For this review, use the dimensioned drawing (mm, ordinates from the lowest corner) and the shaded views. Round coordinates to 2 decimals unless told otherwise and drop trailing zeros. Order: outer loops, then holes, each group sorted by start corner. A loop starts at its lowest first (then second) coordinate and runs counter-clockwise, first axis right, second up. Notation, with made-up numbers: (59.5, 6) - (103.5, 6) arc R21 cw to (103.5, 32) - close; hole circle Ø3 at (62, 2.25). An arc over 180 degrees is marked (long way). Write each question's results on one line, items separated by ' | '. Start each with the question number.
(1) Take a section at D-D, the plane z = 4. Give the boundary of the cut face in (x, y), plus the area to 3 significant figures.
(2) Take a section at C-C, the plane y = 9. Give the boundary of the cut face in (x, z).
(3) For L1, parallel to Z at x = 38.75, y = 3; L2, parallel to X at y = 4, z = 10; L3, parallel to X at y = 0.75, z = 11, list the stretches that pass through material, from the lowest coordinate up. Write a range as from..to.
(4) Take a section at B-B, the plane z = 10. Give the boundary of the cut face in (x, y), plus the area to 3 significant figures.
(5) Insertion check: pin 1 Ø2 at (y, z) = (11, 14.5) entering from -X (3 decimals); pin 2 Ø4 at (y, z) = (7.5, 12) entering from -X; pin 3 Ø4 at (y, z) = (2, 17.5) entering from +X (3 decimals). Each pin has a flat end and moves straight along its axis. Give the tip position at first contact, or say it passes through.
(6) Draft analysis for pull direction X (two halves, no side actions). For the marked faces 1, 2 and 3, state which applies: pulls with the +X half, pulls with the -X half, needs draft (parallel to the pull), parting line crosses it, or undercut.
(7) Take a section at A-A, the plane x = 13.25. Give the boundary of the cut face in (y, z).
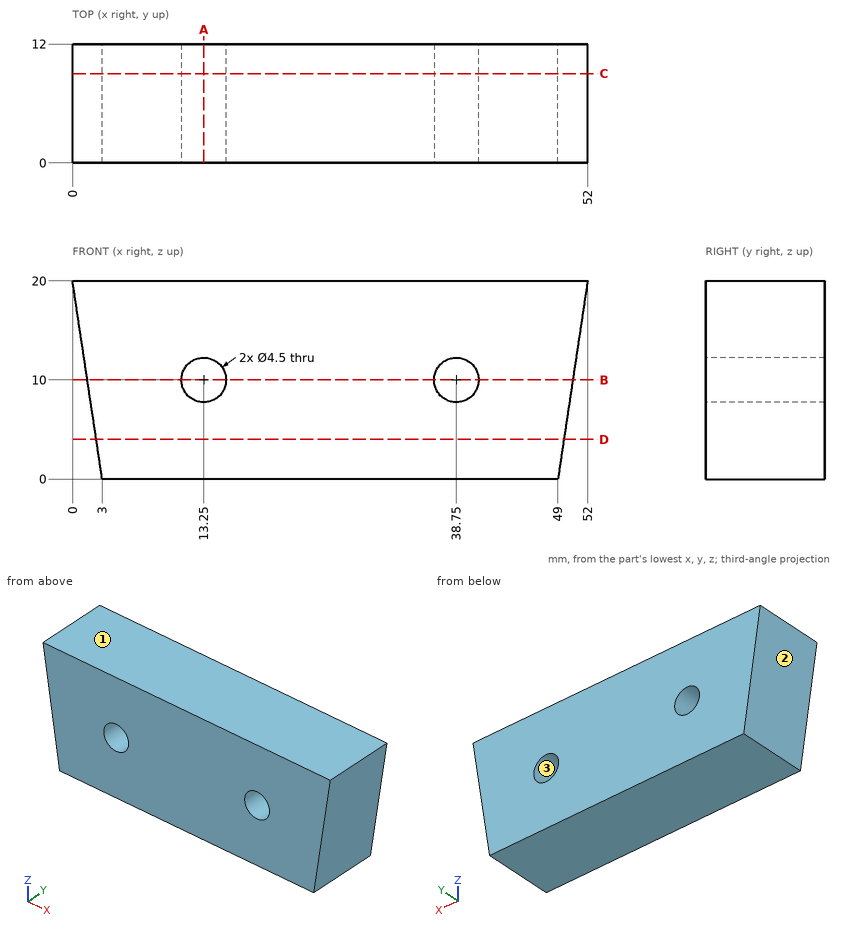
Results below:
1) outline: (2.4, 0) - (49.6, 0) - (49.6, 12) - (2.4, 12) - close | area: 566 mm^2
2) outline: (0, 20) - (3, 0) - (49, 0) - (52, 20) - close; hole circle Ø4.5 at (13.25, 10); hole circle Ø4.5 at (38.75, 10)
3) L1: z = 0..7.75, 12.25..20 | L2: x = 1.5..11, 15.5..36.5, 41..50.5 | L3: x = 1.35..11.23, 15.27..36.73, 40.77..50.65
4) outline: (1.5, 0) - (11, 0) - (11, 12) - (1.5, 12) - close; (15.5, 0) - (36.5, 0) - (36.5, 12) - (15.5, 12) - close; (41, 0) - (50.5, 0) - (50.5, 12) - (41, 12) - close | area: 480 mm^2
5) pin 1: stops at x = 0.675 | pin 2: stops at x = 0.9 | pin 3: stops at x = 51.925
6) face 1: needs draft | face 2: pulls with the -X half | face 3: undercut
7) outline: (0, 0) - (12, 0) - (12, 7.75) - (0, 7.75) - close; (0, 12.25) - (12, 12.25) - (12, 20) - (0, 20) - close
